from build123d import *

# Parameters (mm, degrees)
F0_R     = 6.35
F1_DEPTH = 101.6
F2_R     = 12.7
F3_DEPTH = 12.7
F4_R     = 12.69999


# Not quite as in the source:
# - a fillet or chamfer is up to 0.001 mm smaller than in the source, because OpenCascade refuses the exact size


with BuildPart() as f1:
    # F0 (on Front) → F1 (new body)
    with BuildSketch(Plane.XZ):
        Circle(F0_R)
    extrude(amount=F1_DEPTH)

    # F2 (on Front) → F3 (join)
    with BuildSketch(Plane.XZ):
        Circle(F2_R)
    extrude(amount=F3_DEPTH)

    # F4 (radius 12.7 in the source; OpenCascade refuses exactly that, so slightly less here)
    f4_edges = [f1.edges().sort_by_distance(p)[0] for p in [
        (-12.7, 0, 0),
    ]]
    fillet(f4_edges, radius=F4_R)


solid = f1.part
Geometry: final body of the model. Coordinates: model frame, mm. A direction names the side the tool comes from. Coordinates: 2 decimals unless noted, no trailing zeros. Loops run counter-clockwise (first coordinate to the right, second up) from the corner with the lowest first, then second, coordinate; pieces in that order, holes last. Notation, with made-up numbers: (86, 20) - (105, 20) arc R33 cw to (105, 54) - close; hole circle Ø11 at (4, 80.25). An arc over 180 degrees is marked (long way). Put each result on its own line as item: value. Start each with the question number.
Q1. Set-up query: faces 1 (the flat face through (3, -12.7, 6)), 2 (the flat face through (0, -101.6, 0)). Return all of +Z, -Z, +X, -X, +Y, -Y with unobstructed straight access to the full face (end or side cutting, diameter ignored); none if empty.
Q2. Cut plane A-A, the plane y = -52.5. Return loops of the section in (x, z), and give its area (3 significant figures).
Q3. Line query: line 1 (Y direction, x = 8, z = 3); line 2 (Z direction, x = 3.5, y = -11); line 3 (X direction, y = -60, z = -1). Output: solid intervals per line, ascending.
Q4. Pin query (flat end, axial travel): pin 1 Ø1 at (x, z) = (-8.5, 8) entering from -Y; pin 2 Ø3 at (x, z) = (-2, -5) entering from +Y; pin 3 Ø8 at (y, z) = (-72.5, 6.5) entering from -X. Return the tip coordinate at first contact, or that it passes through.
Filled sheet:
1. face 1: -Y
1. face 2: +Z, -Z, +X, -X, -Y
2. outline: circle Ø12.7 at (0, 0)
2. area: 127 mm²
3. line 1: -12.7 to -3.3
3. line 2: -12.09 to 12.09
3. line 3: -6.27 to 6.27
4. pin 1: y = -12.7
4. pin 2: y = -0.61
4. pin 3: x = -5.84
